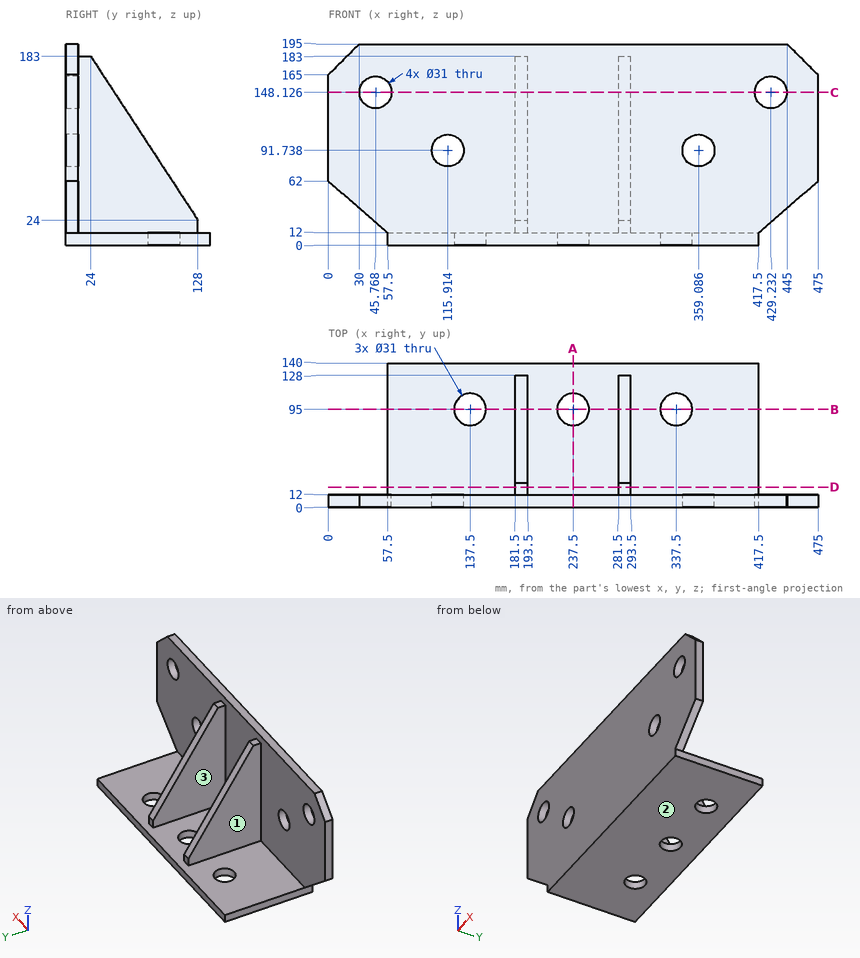
Job drawing, mm, ordinate dimensions from the low corner. One solid piece. A direction names the side the tool comes from. Round coordinates to 2 decimals unless told otherwise and drop trailing zeros. Loops run counter-clockwise (first coordinate to the right, second up) from the corner with the lowest first, then second, coordinate; pieces in that order, holes last.
(1) Cut at A-A (x = 237.5). Give the cut face in (y, z).
(2) Wall check: line 1 along X through (y, z) = (18, 124); line 2 along Y through (x, z) = (237.5, 3.5); line 3 along Y through (x, z) = (331.5, 182.5). Give the ranges that are in metal, low to high.
(3) Cut at B-B (y = 95). Give the cut face in (x, z), plus the area to 3 significant figures.
(4) Cut at C-C (z = 148). Give the cut face in (x, y).
(5) Which spindle directions (+Z, -Z, +X, -X, +Y, -Y) get a long thin tool onto all of the face, cutting with end or side? Do the marked faces 1, 2 and 3. Say none if no direction does.
(6) Drop flat-ended pins along their axis: pin 1 (6 mm diameter, centred on x = 284.5, y = 18.5, fed in from +Z); pin 2 (6 mm diameter, centred on x = 188.5, z = 20, fed in from +Y); pin 3 (4 mm diameter, centred on y = 33.5, z = 54.5, fed in from +X); pin 4 (5 mm diameter, centred on x = 404.5, y = 125, fed in from -Z). Give the stop position or say it passes through.
(7) Cut at D-D (y = 19.5). Give the cut face in (x, z).
Findings below:
1. outline: (0, 0) - (79.5, 0) - (79.5, 12) - (12, 12) - (12, 195) - (0, 195) - close; (110.5, 0) - (140, 0) - (140, 12) - (110.5, 12) - close
2. line 1: x = 181.5 to 193.5, 281.5 to 293.5
2. line 2: y = 0 to 79.5, 110.5 to 140
2. line 3: y = 0 to 12
3. outline: (57.5, 0) - (122, 0) - (122, 12) - (57.5, 12) - close; (153, 0) - (222, 0) - (222, 12) - (193.5, 12) - (193.5, 74.45) - (181.5, 74.45) - (181.5, 12) - (153, 12) - close; (253, 0) - (322, 0) - (322, 12) - (293.5, 12) - (293.5, 74.45) - (281.5, 74.45) - (281.5, 12) - (253, 12) - close; (353, 0) - (417.5, 0) - (417.5, 12) - (353, 12) - close
3. area: 4,700 mm2
4. outline: (0, 0) - (30.27, 0) - (30.27, 12) - (0, 12) - close; (61.27, 0) - (413.73, 0) - (413.73, 12) - (293.5, 12) - (293.5, 46.89) - (281.5, 46.89) - (281.5, 12) - (193.5, 12) - (193.5, 46.89) - (181.5, 46.89) - (181.5, 12) - (61.27, 12) - close; (444.73, 0) - (475, 0) - (475, 12) - (444.73, 12) - close
5. face 1: +Z, -X, +Y
5. face 2: -Z, +X, -X, +Y, -Y
5. face 3: +Z, +Y
6. pin 1: stops at z = 183
6. pin 2: stops at y = 128
6. pin 3: stops at x = 293.5
6. pin 4: stops at z = 0
7. outline: (57.5, 0) - (417.5, 0) - (417.5, 12) - (293.5, 12) - (293.5, 183) - (281.5, 183) - (281.5, 12) - (193.5, 12) - (193.5, 183) - (181.5, 183) - (181.5, 12) - (57.5, 12) - close
